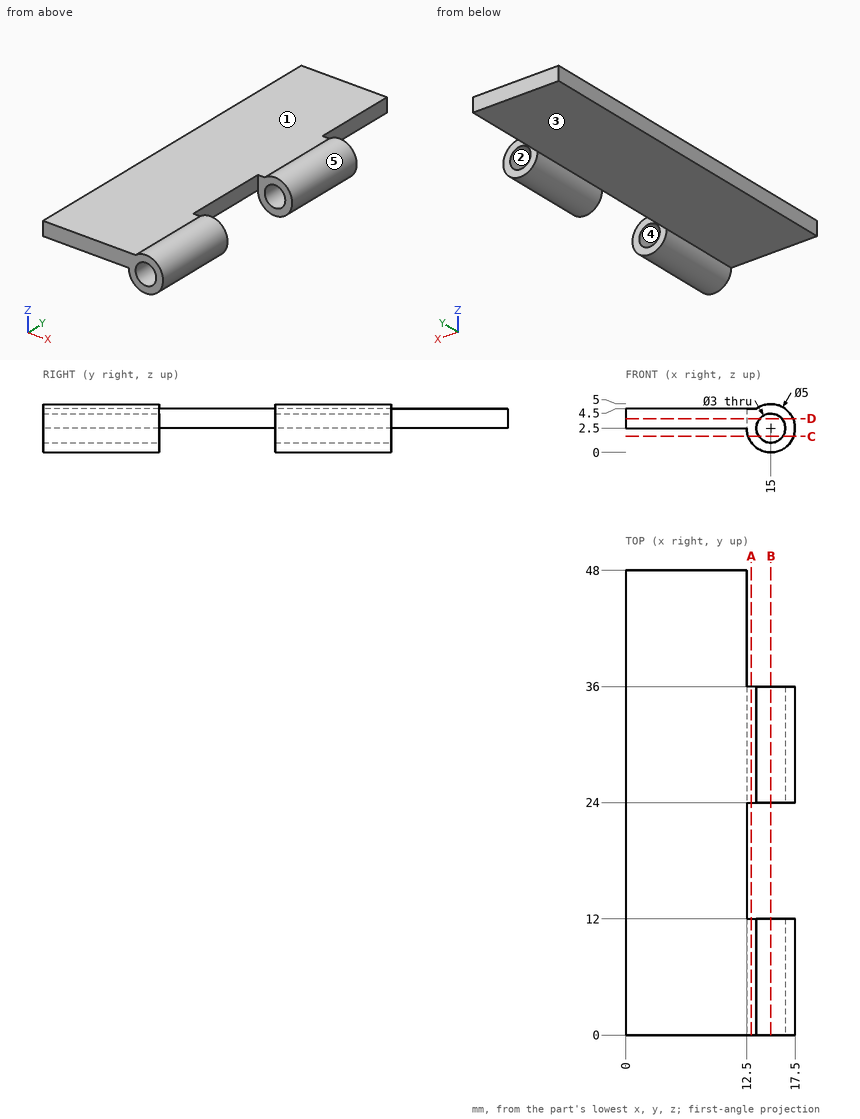
Input: dimensioned drawing with shaded views. Units: mm. Origin: part minimum x, y, z. A direction names the side the tool comes from. Coordinates: 2 decimals unless noted, no trailing zeros. Order: outer loops, then holes, each group sorted by start corner. A loop starts at its lowest first (then second) coordinate and runs counter-clockwise, first axis right, second up.
(1) Access query for the marked faces 1 and 2. Directions: +Z, -Z, +X, -X, +Y, -Y. A direction counts if a zero-diameter tool reaches every point of the face in a straight line with its end or side. Return the directions, or none.
(2) Draft query along Z for the marked faces 3, 4 and 5. Return one class per face: pulls with the +Z half, pulls with the -Z half, needs draft (parallel to the pull), parting line crosses it, or undercut.
(3) Section query C-C (z = 1.65). Return the cut outline in (x, y), plus the area to 3 significant figures.
(4) Section query D-D (z = 3.5). Return the cut outline in (x, y).
(5) Section query A-A (x = 13). Return the cut outline in (y, z), plus the area to 3 significant figures.
(6) Material intervals for probe 1 along Z at (x, y) = (15, 33); probe 2 along Y at (x, z) = (13, 3.8); probe 3 along Z at (x, y) = (9, 14.5), sorted ascending.
(7) Section query B-B (x = 15). Return the cut outline in (y, z).
(8) First-contact query: pin 1 (4 mm diameter, centred on x = 6, y = 20.5, fed in from -Z); pin 2 (4 mm diameter, centred on x = 4, y = 30, fed in from +Z); pin 3 (1.6 mm diameter, centred on y = 17, z = 3.5, fed in from +X); pin 4 (1 mm diameter, centred on x = 5.5, z = 1, fed in from +Y). Flat tips, straight axial feed; report the tip coordinate or a pass-through.
Solution:
1. face 1: +Z, -X, +Y, -Y
1. face 2: +Y, -Y
2. face 3: pulls with the -Z half
2. face 4: undercut
2. face 5: parting line crosses it
3. outline: (12.65, 0) - (13.76, 0) - (13.76, 12) - (12.65, 12) - close; (12.65, 24) - (13.76, 24) - (13.76, 36) - (12.65, 36) - close; (16.24, 0) - (17.35, 0) - (17.35, 12) - (16.24, 12) - close; (16.24, 24) - (17.35, 24) - (17.35, 36) - (16.24, 36) - close
3. area: 53.5 mm2
4. outline: (0, 0) - (13.88, 0) - (13.88, 12) - (12.5, 12) - (12.5, 24) - (13.88, 24) - (13.88, 36) - (12.5, 36) - (12.5, 48) - (0, 48) - close; (16.12, 0) - (17.29, 0) - (17.29, 12) - (16.12, 12) - close; (16.12, 24) - (17.29, 24) - (17.29, 36) - (16.12, 36) - close
5. outline: (0, 1) - (12, 1) - (12, 4.5) - (0, 4.5) - close; (24, 1) - (36, 1) - (36, 4.5) - (24, 4.5) - close
5. area: 84.0 mm2
6. probe 1: z = 0 to 1, 4 to 5
6. probe 2: y = 0 to 12, 24 to 36
6. probe 3: z = 2.5 to 4.5
7. outline: (0, 0) - (12, 0) - (12, 1) - (0, 1) - close; (0, 4) - (12, 4) - (12, 5) - (0, 5) - close; (24, 0) - (36, 0) - (36, 1) - (24, 1) - close; (24, 4) - (36, 4) - (36, 5) - (24, 5) - close
8. pin 1: stops at z = 2.5
8. pin 2: stops at z = 4.5
8. pin 3: stops at x = 12.5
8. pin 4: passes through
